from build123d import *

# Parameters (mm, degrees)
SKETCH1_R           = 19.84375
BOSS_EXTRUDE1_DEPTH = 37.5
SKETCH2_R           = 39.6875
BOSS_EXTRUDE2_DEPTH = 158.75


with BuildPart() as part:
    # Sketch1 → Boss-Extrude1 (new body)
    with BuildSketch(Plane(origin=(0, 0, 0), x_dir=(1, 0, 0), z_dir=(0, 1, 0))):
        with BuildLine():
            Line((-39.6875, 44.371973929), (-39.6875, 294.371973929))
            ThreePointArc((-39.6875, 294.371973929), (0, 334.059473929), (39.6875, 294.371973929))
            Line((39.6875, 294.371973929), (39.6875, 44.371973929))
            ThreePointArc((39.6875, 44.371973929), (0, -59.53125), (-39.6875, 44.371973929))
        make_face()
        with Locations(Location((0, 294.371973929, 0), (0, 0, 270))):
            Circle(SKETCH1_R, mode=Mode.SUBTRACT)
    extrude(amount=BOSS_EXTRUDE1_DEPTH)

    # Sketch2 → Boss-Extrude2 (add)
    with BuildSketch(Plane.XZ):
        with Locations(Location((0, 0, 0), (0, 0, 90))):
            Circle(SKETCH2_R)
    extrude(amount=BOSS_EXTRUDE2_DEPTH)


solid = part.part
Source: CAD feature listing. Evaluate the final solid. Frame: model axes, mm. A direction names the side the tool comes from. Coordinates: 2 decimals unless noted, no trailing zeros. Loops run counter-clockwise (first coordinate to the right, second up) from the corner with the lowest first, then second, coordinate; pieces in that order, holes last. Notation, with made-up numbers: (58.25, 48) - (72.25, 48) arc R23 ccw to (72.25, 85) - close; hole circle Ø1 at (42.5, 35.5). An arc over 180 degrees is marked (long way). One line per item, written item: value. Start each with the question number.
1. Ray query, L1, parallel to Y at x = -9, z = -70; L2, parallel to X at y = 27, z = -136; L3, parallel to X at y = -148, z = 12.5. Return the intervals inside material, ascending.
2. Section D-D (z = -126.5). Return the cut outline in (x, y), and give its area (3 significant figures).
3. Section C-C (y = -87). Return the cut outline in (x, z) (1 decimal).
4. Mould query, pull axis Z, two halves, no side actions, for faces 1 (the cylindrical face through (-0.87, 18.49, -334.05)), 2 (the cylindrical face through (2.01, 18.488, 59.497)), 3 (the cylindrical face through (0.872, 18.488, -314.197)), 4 (the flat face through (39.688, 18, -171)). Classes: pulls with the +Z half, pulls with the -Z half, needs draft (parallel to the pull), parting line crosses it, or undercut.
5. Section A-A (x = 0). Return the cut outline in (y, z).
6. Set-up query: faces 5 (the flat face through (-39.688, 18, -168)), 6 (the flat face through (1, 37.5, -140)), 7 (the cylindrical face through (-11.921, -78.264, 37.855)). Return all of +Z, -Z, +X, -X, +Y, -Y with unobstructed straight access to the full face (end or side cutting, diameter ignored); none if empty.
7. Section B-B (z = 0). Return the cut outline in (x, y).
8. Contact query for flat-ended pins moving along their axis: P1, Ø4, axis at y = 14.5, z = -126.5, coming from the -X side; P2, Ø1.5, axis at x = 40.5, y = 12.5, coming from the -Z side; P3, Ø5, axis at x = -14.5, y = -39.5, coming from the +Z side; P4, Ø1.5, axis at y = -130, z = -42, coming from the -X side. Output: stop coordinate, or through.
Verdict:
1. L1: y = 0 to 37.5
1. L2: x = -39.69 to 39.69
1. L3: x = -37.67 to 37.67
2. outline: (-39.69, 0) - (39.69, 0) - (39.69, 37.5) - (-39.69, 37.5) - close
2. area: 2,980 mm2
3. outline: circle Ø79.4 at (0, 0)
4. face 1: pulls with the -Z half
4. face 2: parting line crosses it
4. face 3: undercut
4. face 4: needs draft
5. outline: (-158.75, -39.69) - (0, -39.69) - (0, -274.53) - (37.5, -274.53) - (37.5, 59.53) - (0, 59.53) - (0, 39.69) - (-158.75, 39.69) - close; (0, -334.06) - (37.5, -334.06) - (37.5, -314.22) - (0, -314.22) - close
6. face 5: -Z, -X, +Y, -Y
6. face 6: +Z, -Z, +X, -X, +Y
6. face 7: -Y
7. outline: (-59.53, 0) - (-39.69, 0) - (-39.69, -158.75) - (39.69, -158.75) - (39.69, 0) - (59.53, 0) - (59.53, 37.5) - (-59.53, 37.5) - close
8. P1: stops at x = -39.69
8. P2: stops at z = -44.32
8. P3: stops at z = 37.83
8. P4: passes through
